from build123d import *

# Parameters (mm, degrees)
SKETCH_1_R          = 6
SKETCH_1_R_2        = 4
EXTRUDE_1_DEPTH     = 60
SKETCH_2_R          = 9
SKETCH_2_R_2        = 4
EXTRUDE_2_DEPTH     = 3
SKETCH_3_R          = 2.05
CUT_EXTRUDE_1_DEPTH = 25


with BuildPart() as part:
    # 草图1 → 凸台-拉伸1 (new body)
    with BuildSketch(Plane.XY):
        Circle(SKETCH_1_R)
        Circle(SKETCH_1_R_2, mode=Mode.SUBTRACT)
    extrude(amount=EXTRUDE_1_DEPTH)

    # 草图2 → 凸台-拉伸2 (add)
    with BuildSketch(Plane.XY.offset(60)):
        Circle(SKETCH_2_R)
        Circle(SKETCH_2_R_2, mode=Mode.SUBTRACT)
    extrude(amount=EXTRUDE_2_DEPTH)

    # 草图3 → 切除-拉伸1 (cut, symmetric)
    with BuildSketch(Plane(origin=(0, 0, 0), x_dir=(1, 0, 0), z_dir=(0, 1, 0))):
        with Locations(Location((0, -15, 0), (0, 0, 270))):
            Circle(SKETCH_3_R)
    extrude(amount=CUT_EXTRUDE_1_DEPTH, both=True, mode=Mode.SUBTRACT)


solid = part.part
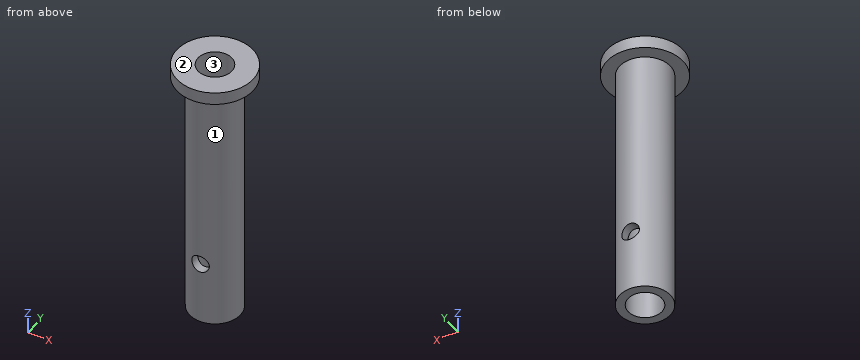
Build history of the part. All positions in model axes, mm. Face numbers are marked on the shaded views. Round coordinates to 2 decimals unless told otherwise and drop trailing zeros. Write each loop counter-clockwise with the first axis right and the second up, starting at its lowest first coordinate (ties: lowest second). Pieces come first, ordered by that corner, then holes. Notation, with made-up numbers: (57, 66) - (85, 66) arc R13 cw to (85, 76) - close; hole circle Ø11 at (85.5, 29). An arc over 180 degrees is marked (long way). One line per question, with ' | ' between items.
1. Mould opens along X. For the marked faces 1, 2 and 3 say: released by +X, released by -X, zero draft, split by the parting line, or undercut.
Results are:
face 1: split by the parting line | face 2: zero draft | face 3: undercut
2. Band-saw the part on A-A, the plane y = 0. Write the cut outline in (x, z).
Results are:
outline: (-9, 60) - (-6, 60) - (-6, 0) - (-4, 0) - (-4, 63) - (-9, 63) - close; (4, 0) - (6, 0) - (6, 60) - (9, 60) - (9, 63) - (4, 63) - close
3. Band-saw the part on D-D, the plane x = -3. Write the cut outline in (y, z).
Results are:
outline: (-8.49, 60) - (-5.2, 60) - (-5.2, 0) - (-2.65, 0) - (-2.65, 63) - (-8.49, 63) - close; (2.65, 0) - (5.2, 0) - (5.2, 60) - (8.49, 60) - (8.49, 63) - (2.65, 63) - close
4. Band-saw the part on B-B, the plane x = 0. Write the cut outline in (y, z).
Results are:
outline: (-9, 60) - (-6, 60) - (-6, 17.05) - (-4, 17.05) - (-4, 63) - (-9, 63) - close; (-6, 0) - (-4, 0) - (-4, 12.95) - (-6, 12.95) - close; (4, 0) - (6, 0) - (6, 12.95) - (4, 12.95) - close; (4, 17.05) - (6, 17.05) - (6, 60) - (9, 60) - (9, 63) - (4, 63) - close
5. Drill centre lines: line 1 along Z through (x, y) = (0, -5); line 2 along Z through (x, y) = (5.5, -6.75); line 3 along X through (y, z) = (5.3, 15). Where is each one in solid material? Low to high. Write a range as from..to.
Results are:
line 1: 0..12.95, 17.05..63 | line 2: 60..63 | line 3: -2.81..-2.05, 2.05..2.81
6. Drop flat-ended pins along their axis: pin 1 Ø6 at (y, z) = (0.5, 55) entering from -X; pin 2 Ø4.5 at (x, z) = (0, 15) entering from -Y; pin 3 Ø6.5 at (x, y) = (0, 0) entering from -Z; pin 4 Ø5 at (y, z) = (4.5, 54.5) entering from -X. Give the stop position or say it passes through.
Results are:
pin 1: x = -6 | pin 2: y = -6 | pin 3: through | pin 4: x = -5.66
7. Band-saw the part on C-C, the plane z = 15. Write the cut outline in (x, y).
Results are:
outline: (-2.05, -5.64) - (-2.05, -3.43) arc R4 cw to (-2.05, 3.43) - (-2.05, 5.64) arc R6 ccw to start; (2.05, -5.64) arc R6 ccw to (2.05, 5.64) - (2.05, 3.43) arc R4 cw to (2.05, -3.43) - close
